from build123d import *

# Parameters (mm, degrees)
CROQUIS1_R              = 5.925
SALIENTE_EXTRUIR1_DEPTH = 9.4
CROQUIS2_R              = 0.25
SALIENTE_EXTRUIR2_DEPTH = 4.9
CROQUIS3_R              = 0.25
SALIENTE_EXTRUIR3_DEPTH = 6.5
CROQUIS4_R              = 1
CORTAR_EXTRUIR1_DEPTH   = 4.5


with BuildPart() as part:
    # Croquis1 → Saliente-Extruir1 (new body)
    with BuildSketch(Plane(origin=(0, 0, 0), x_dir=(1, 0, 0), z_dir=(0, 1, 0))):
        Circle(CROQUIS1_R)
    extrude(amount=SALIENTE_EXTRUIR1_DEPTH)

    # Croquis2 → Saliente-Extruir2 (add)
    with BuildSketch(Plane.XZ):
        with Locations((-3.241786254, 0)):
            Circle(CROQUIS2_R)
    extrude(amount=SALIENTE_EXTRUIR2_DEPTH)

    # Croquis3 → Saliente-Extruir3 (add)
    with BuildSketch(Plane.XZ):
        with Locations((3.241786254, 0)):
            Circle(CROQUIS3_R)
    extrude(amount=SALIENTE_EXTRUIR3_DEPTH)

    # Croquis4 → Cortar-Extruir1 (cut)
    with BuildSketch(Plane(origin=(0, 9.4, 0), x_dir=(1, 0, 0), z_dir=(0, 1, 0))):
        Circle(CROQUIS4_R)
    extrude(amount=-CORTAR_EXTRUIR1_DEPTH, mode=Mode.SUBTRACT)


solid = part.part
Work out the finished part from the listing and answer in its coordinate system (mm). Coordinates: 2 decimals unless noted, no trailing zeros. Order: outer loops, then holes, each group sorted by start corner. A loop starts at its lowest first (then second) coordinate and runs counter-clockwise, first axis right, second up. Notation, with made-up numbers: (53.25, -9.5) - (80.25, -9.5) arc R15 cw to (80.25, 10.5) - close; hole circle Ø9 at (28.5, -25). An arc over 180 degrees is marked (long way). Put each result on its own line as item: value. Start each with the question number.
1) Flat-ended cylindrical pins translate along their axes: pin 1 (2 mm diameter, centred on y = 4.5, z = -3, fed in from +X); pin 2 (1.2 mm diameter, centred on x = 0, z = 0, fed in from +Y); pin 3 (1 mm diameter, centred on x = -3, y = -1.5, fed in from +Z). Find the tip coordinate at first contact, or state that the pin passes through.
2) Find section A-A (x = 0). Give the vertices of the cut face in (y, z) (3 decimals), plus the area to 3 significant figures.
3) Find section C-C (z = 0). Give the vertices of the cut face in (x, y) (3 decimals).
4) Find section D-D (y = -5.5). Give the vertices of the cut face in (x, z).
5) Find the intervals of material crossed by line 1 (X direction, y = 8.35, z = 0) (3 decimals); line 2 (Y direction, x = -0.5, z = -4.25), in increasing order. Write a range as from..to.
6) Find section B-B (y = 6.75). Give the vertices of the cut face in (x, z) (3 decimals), plus the area to 3 significant figures.
7) For a pull along X with two mould halves and no side action, classify faces 1 (the cylindrical face through (5.65, 4.63, -1.78)), 2 (the cylindrical face through (0, 7, 1)), 3 (the flat face through (-0.1, 9.4, 1.2)) as released by +X, released by -X, zero draft, split by the parting line, or undercut.
Results list:
1. pin 1: stops at x = 5.58
1. pin 2: stops at y = 4.9
1. pin 3: stops at z = 0.25
2. outline: (0, -5.925) - (9.4, -5.925) - (9.4, -1) - (4.9, -1) - (4.9, 1) - (9.4, 1) - (9.4, 5.925) - (0, 5.925) - close
2. area: 102 mm^2
3. outline: (-5.925, 0) - (-3.492, 0) - (-3.492, -4.9) - (-2.992, -4.9) - (-2.992, 0) - (2.992, 0) - (2.992, -6.5) - (3.492, -6.5) - (3.492, 0) - (5.925, 0) - (5.925, 9.4) - (1, 9.4) - (1, 4.9) - (-1, 4.9) - (-1, 9.4) - (-5.925, 9.4) - close
4. outline: circle Ø0.5 at (3.24, 0)
5. line 1: x = -5.925..-1, 1..5.925
5. line 2: y = 0..9.4
6. outline: circle Ø11.85 at (0, 0); hole circle Ø2 at (0, 0)
6. area: 107 mm^2
7. face 1: split by the parting line
7. face 2: undercut
7. face 3: zero draft
